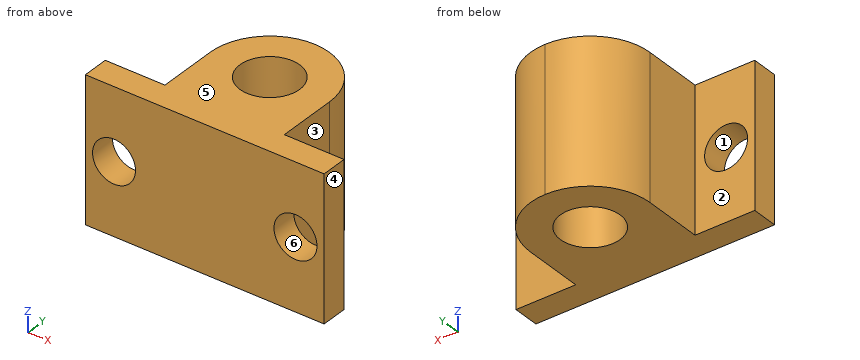
from build123d import *

# Parameters (mm, degrees)
SKETCH1_W           = 25.4
SKETCH1_H           = 15.24
BOSS_EXTRUDE1_DEPTH = 2.794
SKETCH2_W           = 12.7
SKETCH2_H           = 15.24
BOSS_EXTRUDE2_DEPTH = 12.7
FILLET1_R           = 6.35
SKETCH3_R           = 3.175
CUT_EXTRUDE1_DEPTH  = 34.428754628
SKETCH4_R           = 2.286
CUT_EXTRUDE2_DEPTH  = 33.228986953


with BuildPart() as part:
    # Sketch1 → Boss-Extrude1 (new body)
    with BuildSketch(Plane(origin=(0, 0, 0), x_dir=(1, 0, 0), z_dir=(0, 1, 0))):
        with Locations((12.7, 7.62)):
            Rectangle(SKETCH1_W, SKETCH1_H)
    extrude(amount=BOSS_EXTRUDE1_DEPTH)

    # Sketch2 → Boss-Extrude2 (add)
    with BuildSketch(Plane(origin=(0, 2.794, 0), x_dir=(1, 0, 0), z_dir=(0, 1, 0))):
        with Locations((12.7, 7.62)):
            Rectangle(SKETCH2_W, SKETCH2_H)
    extrude(amount=BOSS_EXTRUDE2_DEPTH)

    # Fillet1
    fillet1_edges = [part.edges().sort_by_distance(p)[0] for p in [
        (6.35, 15.494, -7.62),
        (19.05, 15.494, -7.62),
    ]]
    fillet(fillet1_edges, radius=FILLET1_R - 0.0001)  # a hair under: the kernel refuses the full size

    # Sketch3 → Cut-Extrude1 (cut, through all)
    with BuildSketch(Plane.XY):
        with Locations((12.7, 9.144)):
            Circle(SKETCH3_R)
    extrude(amount=-CUT_EXTRUDE1_DEPTH, mode=Mode.SUBTRACT)

    # Sketch4 → Cut-Extrude2 (cut, through all)
    with BuildSketch(Plane(origin=(0, 2.794, 0), x_dir=(1, 0, 0), z_dir=(0, 1, 0))):
        with Locations(Location((3.048, 7.62, 0), (0, 0, 270))):
            Circle(SKETCH4_R)
        with Locations(Location((22.352, 7.62, 0), (0, 0, 270))):
            Circle(SKETCH4_R)
    extrude(amount=-CUT_EXTRUDE2_DEPTH, mode=Mode.SUBTRACT)


solid = part.part
The model under review builds one solid part; all positions refer to its coordinate system, in mm. Face numbers are marked on the shaded views. A direction names the side the tool comes from. Give positions to 0.01 mm unless a question says otherwise; leave off trailing zeros. Write each loop counter-clockwise with the first axis right and the second up, starting at its lowest first coordinate (ties: lowest second). Pieces come first, ordered by that corner, then holes.
1. For P1, Ø1.9, axis at x = 21, z = -6.5, coming from the +Y side; P2, Ø4, axis at x = 3.048, z = -7.62, coming from the +Y side; P3, Ø3, axis at y = 5, z = -9, coming from the -X side; P4, Ø6, axis at y = 8.5, z = -12.5, coming from the +X side, all flat-tipped, find the tip position at first contact; note any pin that passes through.
2. Add section A-A, the plane z = -9. Count the separate pieces of the cut face and the enclosed holes in it, plus the area to 3 significant figures.
3. Tool access review of the marked faces 1, 2 and 3: name each direction out of +Z, -Z, +X, -X, +Y, -Y from which nothing blocks a thin tool from reaching the whole face with its end or side.
4. Add section C-C, the plane y = 8.25. Write out the cut boundary in (x, z).
5. Add section B-B, the plane x = 15.25. Write out the cut boundary in (y, z), plus the area to 3 significant figures.
6. Wall thickness on L1, parallel to X at y = 1.45, z = -7.62; L2, parallel to Y at x = 12.5, z = -4; L3, parallel to X at y = 9.25, z = -6: over which ranges is each line inside the solid? List them lowest first.
7. Draft analysis for pull direction X (two halves, no side actions). For the marked faces 4, 5 and 6, state which applies: +X half, -X half, draft (parallel to the pull), parting line (faces both ways), or undercut.
Worked answers:
1. P1: stops at y = 2.79
1. P2: passes through
1. P3: stops at x = 6.35
1. P4: stops at x = 19.05
2. separate pieces: 3
2. enclosed holes: 1
2. area: 163 mm2
3. face 1: +Y, -Y
3. face 2: +Z, -Z, -X, +Y
3. face 3: +Z, -Z, +X, +Y
4. outline: (6.35, -15.24) - (9.65, -15.24) - (9.65, 0) - (6.35, 0) - close; (15.75, -15.24) - (19.05, -15.24) - (19.05, 0) - (15.75, 0) - close
5. outline: (0, -15.24) - (7.25, -15.24) - (7.25, 0) - (0, 0) - close; (11.04, -15.24) - (14.96, -15.24) - (14.96, 0) - (11.04, 0) - close
5. area: 170 mm2
6. L1: x = 0 to 0.76, 5.33 to 20.07, 24.64 to 25.4
6. L2: y = 0 to 5.98, 12.31 to 15.49
6. L3: x = 6.35 to 9.53, 15.87 to 19.05
7. face 4: +X half
7. face 5: draft
7. face 6: undercut
